```python
from build123d import *

# Parameters (mm, degrees)
F0_W      = 60
F0_H      = 60
F0_W_2    = 43.4
F0_H_2    = 22.4
F0_W_3    = 39.4
F0_H_3    = 18.4
F0_R      = 2
F1_DEPTH  = 2
F2_R      = 1.55
F3_DEPTH  = 2
F4_DEPTH  = 15
F5_R      = 3.5
F7_R      = 3.5
F8_R      = 2
F10_DEPTH = 5


# Not quite as in the source:
# - a pattern or mirror of a feature is missing from the dataset's text; its kind, count and spacing are read off the source's solid
# - a feature names something its author has since deleted; it is built from what else it names


with BuildPart() as f1:
    # F0 (on Top) → F1 (new body)
    with BuildSketch(Plane.XY):
        Rectangle(F0_W, F0_H)
        Rectangle(F0_W_2, F0_H_2, mode=Mode.SUBTRACT)
        Rectangle(F0_W_2, F0_H_2)
        Rectangle(F0_W_3, F0_H_3, mode=Mode.SUBTRACT)
        Rectangle(F0_W_3, F0_H_3)
        with Locations((-10.6629617512, 0)):
            Circle(F0_R, mode=Mode.SUBTRACT)
        with Locations((-10.6629617512, 0)):
            Circle(F0_R)
    extrude(amount=-F1_DEPTH)

    # F2 (on Top) → F3 (join)
    with BuildSketch(Plane.XY):
        Polygon((42.0728534806, 47.0226009489), (-2.4748737342, 2.4748737342), (2.4748737342, -2.4748737342), (47.0226009489, 42.0728534806), align=None)
        Polygon((47.0226009489, 51.9723484172), (42.0728534806, 47.0226009489), (47.0226009489, 42.0728534806), (51.9723484172, 47.0226009489), align=None)
        with Locations((47.0226009489, 47.0226009489)):
            Circle(F2_R, mode=Mode.SUBTRACT)
        with Locations((47.0226009489, 47.0226009489)):
            Circle(F2_R)
    extrude(amount=-F3_DEPTH)

    # F0 (on Top) → F4 (join)
    with BuildSketch(Plane.XY):
        Rectangle(F0_W_2, F0_H_2)
        Rectangle(F0_W_3, F0_H_3, mode=Mode.SUBTRACT)
    extrude(amount=F4_DEPTH)

    # F0 (on Top) → F6 section 0
    with BuildSketch(Plane.XY):
        with Locations((-10.6629617512, 0)):
            Circle(F0_R)
    # F5 (on face) → F6 section 1
    with BuildSketch(Plane(origin=(0, 0, -2), x_dir=(1, 0, 0), z_dir=(0, 0, -1))):
        with Locations((-10.6629617512, 0)):
            Circle(F5_R)
    f6 = loft(mode=Mode.SUBTRACT)

    # F6_copies: F6 across plane
    add(f6.mirror(Plane(origin=(0, 0, 0), x_dir=(0, 0, 1), z_dir=(1, 0, 0))), mode=Mode.SUBTRACT)

    # F7 (on face) → F9 section 0
    with BuildSketch(Plane.XZ.offset(11.2)):
        with Locations((0, 7.5)):
            Circle(F7_R)
    # F8 (on face) → F9 section 1
    with BuildSketch(Plane(origin=(0, -9.2, 0), x_dir=(-1, 0, 0), z_dir=(0, 1, 0))):
        with Locations((0, 7.5)):
            Circle(F8_R)
    loft(mode=Mode.SUBTRACT)

    # F2 (on Top) → F10 (join)
    with BuildSketch(Plane.XY):
        Polygon((47.0226009489, 51.9723484172), (42.0728534806, 47.0226009489), (47.0226009489, 42.0728534806), (51.9723484172, 47.0226009489), align=None)
        with Locations((47.0226009489, 47.0226009489)):
            Circle(F2_R, mode=Mode.SUBTRACT)
    extrude(amount=F10_DEPTH)


solid = f1.part
```
Can you work these out from the model? Positions are in its coordinate system, mm. A direction names the side the tool comes from. Round coordinates to 2 decimals unless told otherwise and drop trailing zeros. Loops run counter-clockwise (first coordinate to the right, second up) from the corner with the lowest first, then second, coordinate; pieces in that order, holes last. Notation, with made-up numbers: (36.25, 36) -> (58.25, 36) arc R23 ccw to (58.25, 47) -> close; hole circle Ø4 at (46, -30). An arc over 180 degrees is marked (long way). Answer in a Markdown table with one row per item.
Item 1: On a 3-axis mill with a long thin cutter (end or side, diameter ignored), from which of +Z, -Z, +X, -X, +Y, -Y can I reach the whole of each face in a straight line? I mean faces 1 (the flat face through (-3, 30, -1)), 2 (the flat face through (44.513, 44.582, 2.465)), 3 (the flat face through (0, 11.2, 7)), 4 (the flat face through (-19.7, 0, 7)), 5 (the flat face through (30, -3, -1)). Say none if no direction works.
Answer block:
| item | result |
|---|---|
| face 1 | +Z, -Z, -X, +Y |
| face 2 | +Z, -X, -Y |
| face 3 | +Z, +X, -X, +Y |
| face 4 | +Z |
| face 5 | +Z, -Z, +X, -Y |
Item 2: We'd pull the mould along X, two halves only. Please class faces 6 (the flat face through (-21.7, 0, 7)), 7 (the cylindrical face through (45.474, 47.091, 2.465)), 8 (the flat face through (0, 0, 0)), 9 (the flat face through (-5, -11.2, 7)): released by +X, released by -X, zero draft, split by the parting line, or undercut.
Answer block:
| item | result |
|---|---|
| face 6 | released by -X |
| face 7 | undercut |
| face 8 | undercut |
| face 9 | zero draft |
Item 3: If I drill on probe 1 along Y at (x, z) = (-3.5, 8.5); probe 2 along Z at (x, y) = (-16, 3.5); probe 3 along X at (y, z) = (11, 8.5), over which ranges is the centre line in solid material (lowest first)?
Answer block:
| item | result |
|---|---|
| probe 1 | -11.2 to -9.2, 9.2 to 11.2 |
| probe 2 | -2 to 0 |
| probe 3 | -21.7 to 21.7 |
Item 4: Suppose I cut it at C-C, the plane y = 8. List the corners of the cut face in (x, z) for me, plus the area to 3 significant figures.
Answer block:
| item | result |
|---|---|
| outline | (-30, -2) -> (30, -2) -> (30, 0) -> (21.7, 0) -> (21.7, 15) -> (19.7, 15) -> (19.7, 0) -> (-19.7, 0) -> (-19.7, 15) -> (-21.7, 15) -> (-21.7, 0) -> (-30, 0) -> close |
| area | 180 mm² |
Item 5: Suppose I cut it at D-D, the plane x = 43.5. List the corners of the cut face in (y, z) for me, plus the area to 3 significant figures.
Answer block:
| item | result |
|---|---|
| outline | (38.55, -2) -> (48.45, -2) -> (48.45, 5) -> (45.6, 5) -> (45.6, 0) -> (38.55, 0) -> close |
| area | 34.1 mm² |
Item 6: Suppose I cut it at A-A, the plane z = 2.5. List the corners of the cut face in (x, y) for me.
Answer block:
| item | result |
|---|---|
| outline | (-21.7, -11.2) -> (21.7, -11.2) -> (21.7, 11.2) -> (-21.7, 11.2) -> close; (42.07, 47.02) -> (47.02, 42.07) -> (51.97, 47.02) -> (47.02, 51.97) -> close; hole (-19.7, -9.2) -> (19.7, -9.2) -> (19.7, 9.2) -> (-19.7, 9.2) -> close; hole circle Ø3.1 at (47.02, 47.02) |
Item 7: Will these pins go through, and if not, where does the flat tip stop? P1, Ø1.5, axis at x = 47, y = 46.5, coming from the +Z side; P2, Ø4.5, axis at x = -10, z = 4, coming from the +Y side; P3, Ø10, axis at x = 1.5, z = 2, coming from the -Y side; P4, Ø6, axis at y = 40, z = 1, coming from the -X side.
Answer block:
| item | result |
|---|---|
| P1 | z = 0 |
| P2 | y = 11.2 |
| P3 | y = -30 |
| P4 | x = 32.22 |
Item 8: Suppose I cut it at B-B, the plane x = 0. List the corners of the cut face in (y, z) for me, plus the area to 3 significant figures.
Answer block:
| item | result |
|---|---|
| outline | (-30, -2) -> (30, -2) -> (30, 0) -> (11.2, 0) -> (11.2, 15) -> (9.2, 15) -> (9.2, 0) -> (-9.2, 0) -> (-9.2, 5.5) -> (-11.2, 4) -> (-11.2, 0) -> (-30, 0) -> close; (-11.2, 11) -> (-9.2, 9.5) -> (-9.2, 15) -> (-11.2, 15) -> close |
| area | 169 mm² |
